Verification items for the finished model (mm, model axes). Coordinates: 2 decimals unless noted, no trailing zeros. Write each loop counter-clockwise with the first axis right and the second up, starting at its lowest first coordinate (ties: lowest second). Pieces come first, ordered by that corner, then holes. Notation, with made-up numbers: (77, -13.5) -> (123, -13.5) arc R27 cw to (123, 6.5) -> close; hole circle Ø10 at (72.25, 87.5). An arc over 180 degrees is marked (long way). Answer in a Markdown table with one row per item.
```python
from build123d import *

# Parameters (mm, degrees)
SKETCH_1_R      = 1.625
SKETCH_1_R_2    = 1.5
EXTRUDE_1_DEPTH = 5
CHAMFER_1_SIZE  = 0.5
EXTRUDE_2_DEPTH = 5


with BuildPart() as part:
    # 草图1 → 凸台-拉伸1 (new body)
    with BuildSketch(Plane(origin=(2.5, 0, 0), x_dir=(0, 0, -1), z_dir=(1, 0, 0))):
        with BuildLine():
            Line((-28.835359751, 3.5), (-97.743384645, 3.5))
            ThreePointArc((-97.743384645, 3.5), (-99.985771473, 3.626105029), (-102.199880675, 4.002829869))
            Line((-102.199880675, 4.002829869), (-115.300119325, 6.997170131))
            ThreePointArc((-115.300119325, 6.997170131), (-117.514228527, 7.373894971), (-119.756615355, 7.5))
            Line((-119.756615355, 7.5), (-125, 7.5))
            ThreePointArc((-125, 7.5), (-132.404899181, 1.190574699), (-127.350956164, -7.122008503))
            Line((-127.350956164, -7.122008503), (-108.053575901, -13.492022674))
            ThreePointArc((-108.053575901, -13.492022674), (-104.959225327, -14.246397817), (-101.784359462, -14.5))
            Line((-101.784359462, -14.5), (-13.675, -14.5))
            Line((-13.675, -14.5), (0, -12.5))
            ThreePointArc((0, -12.5), (12.276307634, 2.354202809), (-4.624146867, 11.613236661))
            Line((-4.624146867, 11.613236661), (-21.436724763, 4.918821342))
            ThreePointArc((-21.436724763, 4.918821342), (-25.068635256, 3.857907785), (-28.835359751, 3.5))
        make_face()
        with Locations(Location((-125, 0, 0), (0, 0, 180))):
            Circle(SKETCH_1_R, mode=Mode.SUBTRACT)
        with Locations(Location((-97.5, -5.5, 0), (0, 0, 180))):
            Circle(SKETCH_1_R_2, mode=Mode.SUBTRACT)
        with Locations(Location((-20, -5.5, 0), (0, 0, 180))):
            Circle(SKETCH_1_R_2, mode=Mode.SUBTRACT)
        with Locations(Location((0, 0, 0), (0, 0, 180))):
            Circle(SKETCH_1_R, mode=Mode.SUBTRACT)
        with BuildLine():
            Line((-87.5, -4), (-32.5, -4))
            ThreePointArc((-32.5, -4), (-31, -5.5), (-32.5, -7))
            Line((-32.5, -7), (-87.5, -7))
            ThreePointArc((-87.5, -7), (-89, -5.5), (-87.5, -4))
        make_face(mode=Mode.SUBTRACT)
    extrude(amount=-EXTRUDE_1_DEPTH)

    # 倒角1
    chamfer_1_edges = [part.edges().sort_by_distance(p)[0] for p in [
        (-2.5, 3.626105029, 99.985771473),
        (2.5, 8.266029002, 13.030435815),
        (2.5, 2.354202809, -12.276307634),
        (2.5, -13.5, 6.8375),
        (2.5, -14.5, 57.729679731),
        (2.5, -14.246397817, 104.959225327),
        (2.5, -10.307015588, 117.702266032),
        (2.5, 1.190574699, 132.404899181),
        (2.5, 7.5, 122.378307678),
        (2.5, 7.373894971, 117.514228527),
        (2.5, 5.5, 108.75),
        (-2.5, 5.5, 108.75),
        (2.5, 3.626105029, 99.985771473),
        (2.5, 3.5, 63.289372198),
        (2.5, 3.857907785, 25.068635256),
        (-2.5, 7.373894971, 117.514228527),
        (-2.5, 7.5, 122.378307678),
        (-2.5, 1.190574699, 132.404899181),
        (-2.5, -10.307015588, 117.702266032),
        (-2.5, 0, 123.375),
        (2.5, 0, 123.375),
        (-2.5, -14.246397817, 104.959225327),
        (-2.5, -5.5, 96),
        (2.5, -5.5, 96),
        (-2.5, -5.5, 18.5),
        (-2.5, -14.5, 57.729679731),
        (2.5, -5.5, 18.5),
        (-2.5, -13.5, 6.8375),
        (-2.5, -5.5, 89),
        (-2.5, -4, 60),
        (-2.5, -5.5, 31),
        (-2.5, -7, 60),
        (-2.5, 2.354202809, -12.276307634),
        (2.5, -5.5, 89),
        (2.5, -7, 60),
        (2.5, -5.5, 31),
        (2.5, -4, 60),
        (-2.5, 3.857907785, 25.068635256),
        (-2.5, 8.266029002, 13.030435815),
        (-2.5, 0, -1.625),
        (2.5, 0, -1.625),
        (-2.5, 3.5, 63.289372198),
    ]]
    chamfer(chamfer_1_edges, length=CHAMFER_1_SIZE)

    # Sketch 3D_1 → 凸台-拉伸2 (add)
    with BuildSketch(Plane(origin=(2.5, 0.724565904, 106.04601189), x_dir=(0, -0.10344866174004491, -0.9946347944769446), z_dir=(-1, 0, 0))):
        Polygon((0, 0), (92.493650367, -9.619957398), (96.694027737, 0), (73.434795042, 4.428728496), (1.034783284, 9.949200326), align=None)
    extrude(amount=EXTRUDE_2_DEPTH)


solid = part.part
```
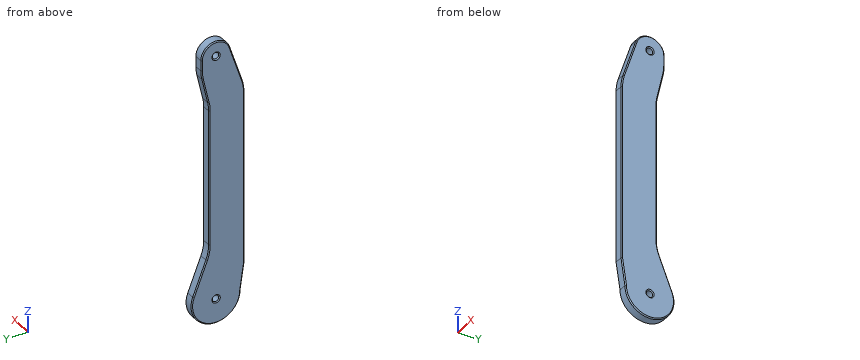
1. Section check A-A, the plane y = 0. Record the boundary of the cut face in (x, z) (3 decimals).
Geometry says:
| item | result |
|---|---|
| outline | (-2.5, -12) -> (-2, -12.5) -> (2, -12.5) -> (2.5, -12) -> (2.5, -2.125) -> (2, -1.625) -> (-2, -1.625) -> (-2.5, -2.125) -> close; (-2.5, 2.125) -> (-2, 1.625) -> (2, 1.625) -> (2.5, 2.125) -> (2.5, 122.875) -> (2, 123.375) -> (-2, 123.375) -> (-2.5, 122.875) -> close; (-2.5, 127.125) -> (-2, 126.625) -> (2, 126.625) -> (2.5, 127.125) -> (2.5, 132) -> (2, 132.5) -> (-2, 132.5) -> (-2.5, 132) -> close |
2. Section check C-C, the plane z = 65. Record the boundary of the cut face in (x, y), plus the area to 3 significant figures.
Geometry says:
| item | result |
|---|---|
| outline | (-2.5, -14) -> (-2, -14.5) -> (2, -14.5) -> (2.5, -14) -> (2.5, 3) -> (2, 3.5) -> (-2, 3.5) -> (-2.5, 3) -> close |
| area | 89.5 mm^2 |
3. Section check D-D, the plane z = 10. Record the boundary of the cut face in (x, y), plus the area to 3 significant figures.
Geometry says:
| item | result |
|---|---|
| outline | (-2.5, -13.46) -> (-2, -13.96) -> (2, -13.96) -> (2.5, -13.46) -> (2.5, 8.93) -> (2, 9.47) -> (-2, 9.47) -> (-2.5, 8.93) -> close |
| area | 117 mm^2 |
4. Thickness scan on line 1 (Z direction, x = 2.05, y = -0.25); line 2 (Z direction, x = -0.95, y = 0.75); line 3 (Y direction, x = -1.9, z = 68). Record the ranges inside material, lowest first. Write a range as from..to.
Geometry says:
| item | result |
|---|---|
| line 1 | -12.45..-1.66, 1.66..123.34, 126.66..132.45 |
| line 2 | -12.48..-1.44, 1.44..123.56, 126.44..132.46 |
| line 3 | -14.5..3.5 |
5. Depth check by flat-ended pin: P1, Ø3, axis at x = -0.5, z = 70, coming from the +Y side; P2, Ø3.5, axis at y = 0, z = 0, coming from the +X side (3 decimals); P3, Ø1.5, axis at x = 1.5, y = -5, coming from the +Z side; P4, Ø1.9, axis at y = 0, z = 125, coming from the -X side. Enter the tip coordinate at first touch or a pass-through.
Geometry says:
| item | result |
|---|---|
| P1 | y = 3.5 |
| P2 | x = 2.125 |
| P3 | z = 131.18 |
| P4 | through |
6. Section check B-B, the plane x = 0.65. Record the boundary of the cut face in (y, z) (3 decimals).
Geometry says:
| item | result |
|---|---|
| outline | (-14.5, 13.675) -> (-12.5, 0) arc R12.5 ccw (long way) to (11.613, 4.624) -> (4.919, 21.437) arc R20 cw to (3.5, 28.835) -> (3.5, 97.743) arc R20 cw to (4.003, 102.2) -> (6.997, 115.3) arc R20 ccw to (7.5, 119.757) -> (7.5, 125) arc R7.5 ccw to (-7.122, 127.351) -> (-13.492, 108.054) arc R20 ccw to (-14.5, 101.784) -> close; hole circle Ø3.25 at (0, 0); hole circle Ø3.25 at (0, 125) |
